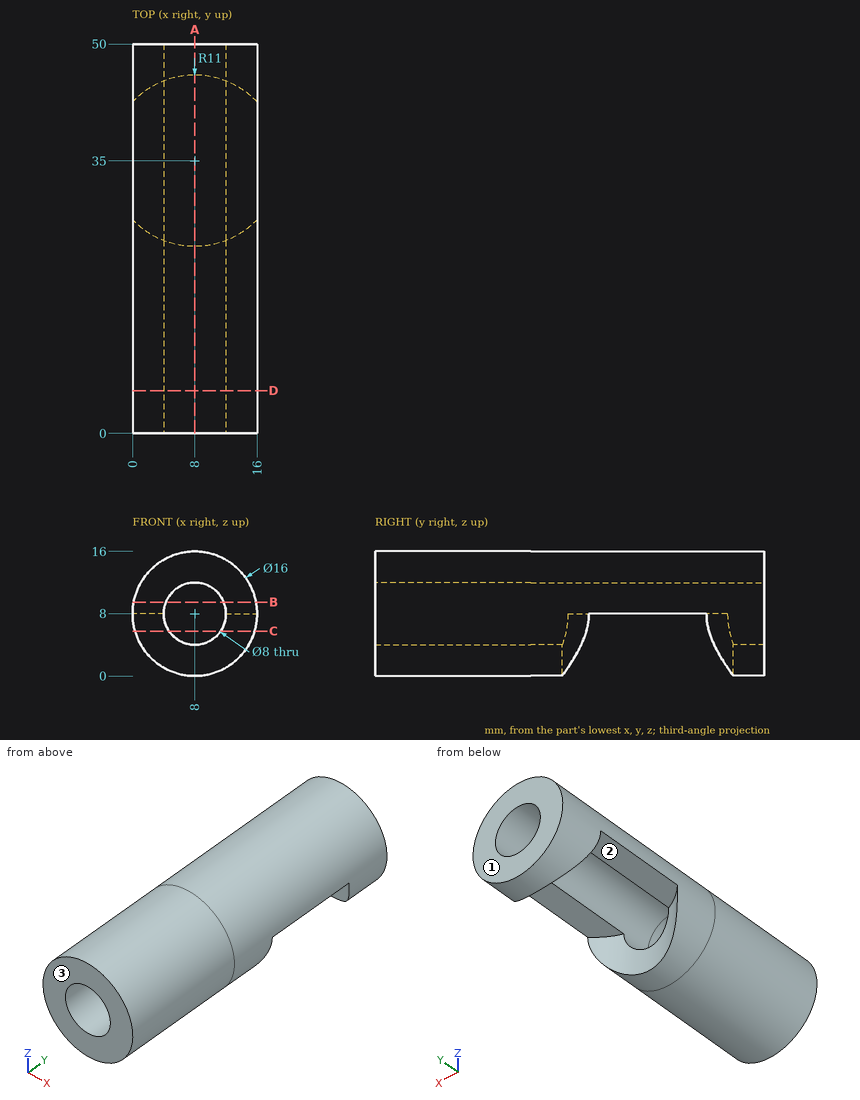
The figure shows three views and two pictorial views of one solid part (mm, origin at its lowest corner). Answer the questions. Give positions to 0.01 mm unless a question says otherwise; leave off trailing zeros. Write each loop counter-clockwise with the first axis right and the second up, starting at its lowest first coordinate (ties: lowest second). Pieces come first, ordered by that corner, then holes. Notation, with made-up numbers: (46.25, 52.5) -> (95.25, 52.5) arc R24 ccw to (95.25, 70.5) -> close; hole circle Ø5 at (63, -22). An arc over 180 degrees is marked (long way). Write each question's results on one line, items separated by ' | '.
1. Determine the mould class of the marked faces 1, 2 and 3 for opening direction Y: +Y half, -Y half, draft (parallel to the pull), parting line (faces both ways), or undercut.
Data:
face 1: +Y half | face 2: undercut | face 3: -Y half
2. Each of these flat-tipped pins is pushed along its axis until it touches: pin 1 Ø4.5 at (x, y) = (14.5, 31) entering from -Z; pin 2 Ø6 at (x, y) = (13.5, 36.5) entering from +Z; pin 3 Ø2 at (y, z) = (28.5, 11) entering from -X. Where does it stop, or does it pass through?
Data:
pin 1: z = 8 | pin 2: z = 15.6 | pin 3: x = 0.25
3. Find section D-D on y = 5.5. Determine the outline of the cut face in (x, z).
Data:
outline: circle Ø16 at (8, 8); hole circle Ø8 at (8, 8)
4. Find section B-B on z = 9.5. Determine the outline of the cut face in (x, y), and give its area (3 significant figures).
Data:
outline: (0.14, 0) -> (4.29, 0) -> (4.29, 50) -> (0.14, 50) -> close; (11.71, 0) -> (15.86, 0) -> (15.86, 50) -> (11.71, 50) -> close | area: 415 mm^2
5. Find section C-C on z = 5.75. Determine the outline of the cut face in (x, y).
Data:
outline: (0.32, 0) -> (4.69, 0) -> (4.69, 24.51) arc R11 cw to (0.32, 27.12) -> close; (0.32, 42.88) arc R11 cw to (4.69, 45.49) -> (4.69, 50) -> (0.32, 50) -> close; (11.31, 0) -> (15.68, 0) -> (15.68, 27.12) arc R11 cw to (11.31, 24.51) -> close; (11.31, 45.49) arc R11 cw to (15.68, 42.88) -> (15.68, 50) -> (11.31, 50) -> close
6. Straight lines are drawn through the part: L1, parallel to X at y = 10.5, z = 8; L2, parallel to X at y = 40.5, z = 9.5; L3, parallel to Y at x = 9, z = 1.5. For each, find the intervals that lie inside material, in ascending order.
Data:
L1: 0 to 4, 12 to 16 | L2: 0.14 to 4.29, 11.71 to 15.86 | L3: 0 to 24.05, 45.95 to 50
7. Find section A-A on x = 8. Determine the outline of the cut face in (y, z).
Data:
outline: (0, 0) -> (24, 0) -> (24, 4) -> (0, 4) -> close; (0, 12) -> (50, 12) -> (50, 16) -> (0, 16) -> close; (46, 0) -> (50, 0) -> (50, 4) -> (46, 4) -> close
